```python
from build123d import *

# Parameters (mm, degrees)
SKETCH1_R               = 12.5
BOSS_EXTRUDE1_DEPTH     = 5
EXTRUDE_THIN1_DEPTH     = 5
SKETCH6_W               = 56.5
SKETCH6_H               = 12.459935794
BOSS_EXTRUDE3_DEPTH     = 5
SKETCH7_R               = 3.25
CUT_EXTRUDE3_DEPTH      = 1
CUT_EXTRUDE3_DEPTH_BACK = 6
BOSS_EXTRUDE4_DEPTH     = 5
SKETCH9_4_W             = 9.626496109
SKETCH9_4_H             = 23.122525611
CUT_EXTRUDE5_DEPTH      = 6
BOSS_EXTRUDE5_DEPTH     = 5
SKETCH11_R              = 2.075
CUT_EXTRUDE6_DEPTH      = 6
SKETCH12_R              = 2.075
CUT_EXTRUDE7_DEPTH      = 6
SKETCH13_R              = 2.075
CUT_EXTRUDE8_DEPTH      = 6
CIRPATTERN1_COUNT       = 6
CIRPATTERN1_ANGLE       = 100
CIRPATTERN2_COUNT       = 6
CIRPATTERN2_ANGLE       = 100
CIRPATTERN3_COUNT       = 6
CIRPATTERN3_ANGLE       = 100
FILLET2_R               = 4


with BuildPart() as part:
    # Sketch1 → Boss-Extrude1 (new body)
    with BuildSketch(Plane(origin=(0, 0, 0), x_dir=(1, 0, 0), z_dir=(0, 1, 0))):
        Circle(SKETCH1_R)
    extrude(amount=BOSS_EXTRUDE1_DEPTH)



with BuildPart() as body_2:
    # Sketch4 → Extrude-Thin1 (new body)
    with BuildSketch(Plane(origin=(0, 0, 0), x_dir=(1, 0, 0), z_dir=(0, 1, 0))):
        with BuildLine():
            ThreePointArc((16.811373022, -54.987523468), (46.221769485, -34.202310238), (57.5, 0))
            Line((57.5, 0), (42.5, 0))
            ThreePointArc((42.5, 0), (34.163916576, -25.279968437), (12.425797451, -40.642952128))
            Line((12.425797451, -40.642952128), (16.811373022, -54.987523468))
        make_face()
    extrude(amount=EXTRUDE_THIN1_DEPTH)


with BuildPart() as part_1:
    add(part.part)

    add(body_2.part)  # Boss-Extrude3 merges body 2
    # Sketch6 → Boss-Extrude3 (add)
    with BuildSketch(Plane(origin=(0, 0, 0), x_dir=(1, 0, 0), z_dir=(0, 1, 0))):
        with Locations((29.25, 6.229967897)):
            Rectangle(SKETCH6_W, SKETCH6_H)
    extrude(amount=BOSS_EXTRUDE3_DEPTH)

    # Sketch7 → Cut-Extrude3 (cut, two sides)
    with BuildSketch(Plane(origin=(0, 5, 0), x_dir=(1, 0, 0), z_dir=(0, 1, 0))) as cut_extrude3_sk:
        Circle(SKETCH7_R)
    extrude(amount=CUT_EXTRUDE3_DEPTH, mode=Mode.SUBTRACT)
    extrude(cut_extrude3_sk.sketch, amount=-CUT_EXTRUDE3_DEPTH_BACK, mode=Mode.SUBTRACT)

    # Sketch9 → Boss-Extrude4 (add)
    with BuildSketch(Plane(origin=(0, 0, 0), x_dir=(1, 0, 0), z_dir=(0, 1, 0))):
        with BuildLine():
            Line((16.811373022, -54.987523468), (14.618585236, -47.815237798))
            Line((14.618585236, -47.815237798), (14.618585236, -55.610673128))
            ThreePointArc((14.618585236, -55.610673128), (15.718067562, -55.309966119), (16.811373022, -54.987523468))
        make_face()
        with BuildLine():
            Line((14.618585236, -47.815237798), (12.425797451, -40.642952128))
            Line((12.425797451, -40.642952128), (11.862973877, -56.262952738))
            ThreePointArc((11.862973877, -56.262952738), (13.244795598, -55.953779046), (14.618585236, -55.610673128))
            Line((14.618585236, -55.610673128), (14.618585236, -47.815237798))
        make_face()
    extrude(amount=BOSS_EXTRUDE4_DEPTH)

    # Sketch9<4> → Cut-Extrude5 (cut, through all)
    with BuildSketch(Plane(origin=(0, 0, 0), x_dir=(1, 0, 0), z_dir=(0, 1, 0))):
        with Locations((9.805337182, -49.150976699)):
            Rectangle(SKETCH9_4_W, SKETCH9_4_H)
    extrude(amount=CUT_EXTRUDE5_DEPTH, mode=Mode.SUBTRACT)

    # Sketch10 → Boss-Extrude5 (add)
    with BuildSketch(Plane(origin=(0, 0, 0), x_dir=(1, 0, 0), z_dir=(0, 1, 0))):
        with BuildLine():
            Line((-23.827361095, 22.831050419), (-5.931209267, 5.683203326))
            Line((-5.931209267, 5.683203326), (19.532104398, 5.683203326))
            Line((19.532104398, 5.683203326), (31.685950206, 9.219574804))
            ThreePointArc((31.685950206, 9.219574804), (7.85858911, 32.050625223), (-23.827361095, 22.831050419))
        make_face()
    extrude(amount=BOSS_EXTRUDE5_DEPTH)

    # Sketch11 → Cut-Extrude6 (cut, through all)
    with BuildSketch(Plane(origin=(0, 5, 0), x_dir=(1, 0, 0), z_dir=(0, 1, 0))):
        with Locations((-8.29398923, 13.682461133)):
            Circle(SKETCH11_R)
    cut_extrude6 = extrude(amount=-CUT_EXTRUDE6_DEPTH, mode=Mode.SUBTRACT)

    # Sketch12 → Cut-Extrude7 (cut, through all)
    with BuildSketch(Plane(origin=(0, 5, 0), x_dir=(1, 0, 0), z_dir=(0, 1, 0))):
        with Locations((-13.000533094, 17.747848863)):
            Circle(SKETCH12_R)
    cut_extrude7 = extrude(amount=-CUT_EXTRUDE7_DEPTH, mode=Mode.SUBTRACT)

    # Sketch13 → Cut-Extrude8 (cut, through all)
    with BuildSketch(Plane(origin=(0, 5, 0), x_dir=(1, 0, 0), z_dir=(0, 1, 0))):
        with Locations((-18.451858843, 21.060125955)):
            Circle(SKETCH13_R)
    cut_extrude8 = extrude(amount=-CUT_EXTRUDE8_DEPTH, mode=Mode.SUBTRACT)

    # CirPattern1: Cut-Extrude6 ×6 about axis
    cirpattern1_axis = Axis((0, 0, 0), (0, -1, 0))
    for i in range(1, CIRPATTERN1_COUNT):
        add(cut_extrude6.rotate(cirpattern1_axis, i * CIRPATTERN1_ANGLE / (CIRPATTERN1_COUNT - 1)), mode=Mode.SUBTRACT)

    # CirPattern2: Cut-Extrude7 ×6 about axis
    cirpattern2_axis = Axis((0, 0, 0), (0, -1, 0))
    for i in range(1, CIRPATTERN2_COUNT):
        add(cut_extrude7.rotate(cirpattern2_axis, i * CIRPATTERN2_ANGLE / (CIRPATTERN2_COUNT - 1)), mode=Mode.SUBTRACT)

    # CirPattern3: Cut-Extrude8 ×6 about axis
    cirpattern3_axis = Axis((0, 0, 0), (0, -1, 0))
    for i in range(1, CIRPATTERN3_COUNT):
        add(cut_extrude8.rotate(cirpattern3_axis, i * CIRPATTERN3_ANGLE / (CIRPATTERN3_COUNT - 1)), mode=Mode.SUBTRACT)

    # Fillet2
    fillet2_edges = [part_1.edges().sort_by_distance(p)[0] for p in [
        (42.5, 2.5, 0),
        (30.557323181, 2.5, -12.459935794),
        (-9.025515566, 2.5, -8.648125159),
        (-23.827361095, 2.5, -22.831050419),
        (12.5, 2.5, 0),
        (57.5, 2.5, -12.459935794),
    ]]
    fillet(fillet2_edges, radius=FILLET2_R)


solid = part_1.part
```
Here's how the part is built. I have some questions about the finished solid (model axes, mm). A direction names the side the tool comes from. Give positions to 0.01 mm unless a question says otherwise; leave off trailing zeros. Order: outer loops, then holes, each group sorted by start corner. A loop starts at its lowest first (then second) coordinate and runs counter-clockwise, first axis right, second up. Notation, with made-up numbers: (4.5, 36) - (43.5, 36) arc R30 ccw to (43.5, 59) - close; hole circle Ø10 at (6.25, 75). An arc over 180 degrees is marked (long way). Answer as a JSON object with one key per item and string values. Group by question number.
Item 1: Please list where these lines run through material, in increasing order: probe 1 along Z at (x, y) = (-2, 1.05); probe 2 along Z at (x, y) = (3, 2.8); probe 3 along X at (y, z) = (3.55, 4).
Item 2: For P1, Ø10.5, axis at x = 0, z = 0, coming from the +Y side; P2, Ø3.5, axis at x = 9.01, z = -26.51, coming from the -Y side, each with a flat end and sliding along its axis, tell me the tip position at first contact or that it passes through.
Item 3: If we section it at D-D on z = 45: Please give me the cut outline in (x, y).
Item 4: If we section it at A-A on z = -10: Please give me the cut outline in (x, y), and give its area (3 significant figures).
Item 5: If we section it at B-B on x = 46: Please give me the cut outline in (y, z).
Item 6: If we section it at C-C on y = 3.8: Give the number of separate pieces and of enclosed holes in the cut face, and give its area (3 significant figures).
Item 7: If we mould it in two halves opening along Z, with no side actions, what happens to faces 4 (the flat face through (57.5, 2, -4)), 5 (the cylindrical face through (33.729, 2.465, 25.858)), 6 (the cylindrical face through (56.297, 2.535, -11.319))? For each: pulls with the +Z half, pulls with the -Z half, needs draft (parallel to the pull), parting line crosses it, or undercut.
Item 8: Which directions (+Z, -Z, +X, -X, +Y, -Y) give clear straight access to the entire face, cutting with the end or side of a thin tool? Please do faces 1 (the cylindrical face through (13.52, 2.54, 0.87)), 2 (the cylindrical face through (-10.372, 2.465, -8.797)), 3 (the flat face through (43, 2, -12.46)).
Result set:
{
 "1": {"probe 1": "-32.94 to -29.52, -26.46 to -17.44, -13.94 to -2.56, 2.56 to 12.34", "probe 2": "-32.86 to -23.33, -20.57 to -17.81, -13.81 to -1.25, 1.25 to 12.13", "probe 3": "-11.84 to 11.84, 42.29 to 57.36"},
 "2": {"P1": "y = 5", "P2": "through"},
 "3": {"outline": "(14.62, 0) - (35.79, 0) - (35.79, 5) - (14.62, 5) - close"},
 "4": {"outline": "(-10.76, 0) - (10.03, 0) - (10.03, 5) - (-10.76, 5) - close; (14.04, 0) - (17.68, 0) - (17.68, 5) - (14.04, 5) - close; (21.79, 0) - (57.19, 0) - (57.19, 5) - (21.79, 5) - close", "area": "299 mm²"},
 "5": {"outline": "(0, -12.46) - (5, -12.46) - (5, 34.5) - (0, 34.5) - close"},
 "6": {"separate pieces": "1", "enclosed holes": "19", "area": "2,600 mm²"},
 "7": {"face 4": "needs draft", "face 5": "undercut", "face 6": "pulls with the -Z half"},
 "8": {"face 1": "+Y, -Y", "face 2": "-X, +Y, -Y", "face 3": "-Z, +X, +Y, -Y"}
}
